Read the model definition and answer for the solid it produces. Units are mm, in the model's axes. Face numbers are marked on the shaded views. Round coordinates to 2 decimals unless told otherwise and drop trailing zeros. Order: outer loops, then holes, each group sorted by start corner. A loop starts at its lowest first (then second) coordinate and runs counter-clockwise, first axis right, second up. Notation, with made-up numbers: (74, -18) - (105, -18) arc R12 cw to (105, -2) - close; hole circle Ø4 at (58, 79). An arc over 180 degrees is marked (long way). Put each result on its own line as item: value. Start each with the question number.
Q1. Find the intervals of material crossed by line 1 along Y through (x, z) = (18.75, 2.5); line 2 along Z through (x, y) = (14, 0); line 3 along X through (y, z) = (-17, 2.25), in increasing order. Write a range as from..to.
Q2. For a pull along Z with two mould halves and no side action, classify the marked faces 1, 2 and 3 as pulls with the +Z half, pulls with the -Z half, needs draft (parallel to the pull), parting line crosses it, or undercut.
Q3. Section B-B on y = -2 is taken. Give the vertices of the cut face in (x, z).
Q4. Each of these flat-tipped pins is pushed along its axis until it touches: pin 1 Ø3 at (y, z) = (19.5, 2.5) entering from +X; pin 2 Ø1.5 at (y, z) = (-19.5, 2.5) entering from -X. Where does it stop, or does it pass through?
Q5. Section A-A on x = 14 is taken. Give the vertices of the cut face in (y, z), then the cut area to 4 significant figures.
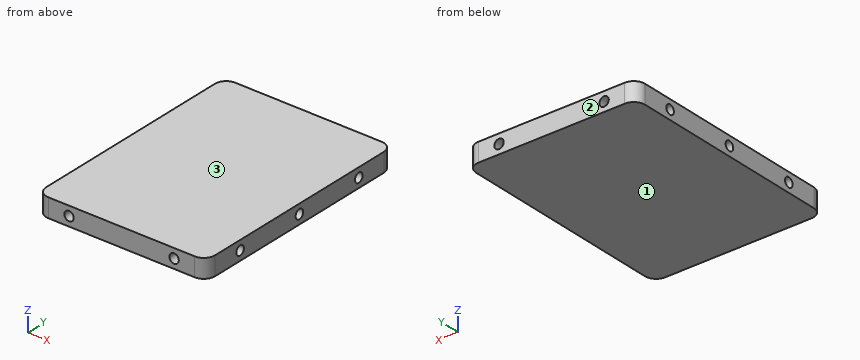
from build123d import *

# Parameters (mm, degrees)
SKETCH_1_W         = 45
SKETCH_1_H         = 61.4
EXTRUDE_1_DEPTH    = 5
HOLE_WIZARD_M3_3_D = 2.5
HOLE_WIZARD_M3_4_D = 2.5
FILLET_1_R         = 3


with BuildPart() as part:
    # 草图1 → 凸台-拉伸1 (new body)
    with BuildSketch(Plane.XY):
        Rectangle(SKETCH_1_W, SKETCH_1_H)
    extrude(amount=EXTRUDE_1_DEPTH)

    # 草图3 → M3 螺纹孔1 (revolve, cut)
    with BuildSketch(Plane(origin=(-22.5, 0, 2.5), x_dir=(0, 0, 1), z_dir=(0, 1, 0))):
        Polygon((0, 0), (0, 5.751075774), (1.25, 5), (1.25, 0), align=None)
    hole_wizard_m3_1 = revolve(axis=Axis((-28.85, 0, 2.5), (1, 0, 0)), mode=Mode.SUBTRACT)

    # 草图5 → M3 螺纹孔2 (revolve, cut)
    with BuildSketch(Plane(origin=(-22.5, 19.5, 2.5), x_dir=(0, 0, 1), z_dir=(0, 1, 0))):
        Polygon((0, 0), (0, 5.751075774), (1.25, 5), (1.25, 0), align=None)
    hole_wizard_m3_2 = revolve(axis=Axis((-28.85, 19.5, 2.5), (1, 0, 0)), mode=Mode.SUBTRACT)

    # 镜向1: M3 螺纹孔2 across plane
    add(hole_wizard_m3_2.mirror(Plane.ZX), mode=Mode.SUBTRACT)

    # M3 螺纹孔3 (through all)
    with Locations(Plane(origin=(0, -30.7, 0), x_dir=(-1, 0, 0), z_dir=(0, -1, 0))):
        with Locations((-14, -2.5)):
            hole_wizard_m3_3 = Hole(HOLE_WIZARD_M3_3_D / 2)

    # 镜向2: M3 螺纹孔3 across plane
    add(hole_wizard_m3_3.mirror(Plane(origin=(0, 0, 0), x_dir=(0, 0, 1), z_dir=(1, 0, 0))), mode=Mode.SUBTRACT)

    # 镜向3: M3 螺纹孔2, M3 螺纹孔1 across plane
    add(hole_wizard_m3_2.mirror(Plane(origin=(0, 0, 0), x_dir=(0, 0, 1), z_dir=(1, 0, 0))), mode=Mode.SUBTRACT)
    add(hole_wizard_m3_1.mirror(Plane(origin=(0, 0, 0), x_dir=(0, 0, 1), z_dir=(1, 0, 0))), mode=Mode.SUBTRACT)

    # 镜向3 copy 1 sketch → 镜向3 copy 1 (revolve, cut)
    with BuildSketch(Plane(origin=(22.5, -19.5, 2.5), x_dir=(0, 0, 1), z_dir=(0, -1, 0))):
        Polygon((0, 0), (0, 5.751075774), (1.25, 5), (1.25, 0), align=None)
    revolve(axis=Axis((28.85, -19.5, 2.5), (-1, 0, 0)), mode=Mode.SUBTRACT)

    # M3 螺纹孔4 (through all)
    with Locations(Plane(origin=(0, 30.7, 0), x_dir=(1, 0, 0), z_dir=(0, 1, 0))):
        with Locations((-14, -2.5), (14, -2.5)):
            Hole(HOLE_WIZARD_M3_4_D / 2)

    # 圆角1
    fillet_1_edges = [part.edges().sort_by_distance(p)[0] for p in [
        (22.5, -30.7, 2.5),
        (-22.5, -30.7, 2.5),
        (-22.5, 30.7, 2.5),
        (22.5, 30.7, 2.5),
    ]]
    fillet(fillet_1_edges, radius=FILLET_1_R)


solid = part.part
Findings:
1. line 1: -30.7..-20.75, -18.25..-1.25, 1.25..18.25, 20.75..30.7
1. line 2: 0..1.25, 3.75..5
1. line 3: -22.5..-15.22, -12.78..12.78, 15.22..22.5
2. face 1: pulls with the -Z half
2. face 2: needs draft
2. face 3: pulls with the +Z half
3. outline: (-22.5, 0) - (22.5, 0) - (22.5, 5) - (-22.5, 5) - close; hole circle Ø2.5 at (-14, 2.5); hole circle Ø2.5 at (14, 2.5)
4. pin 1: x = 22.5
4. pin 2: x = -17.2
5. outline: (-30.7, 0) - (30.7, 0) - (30.7, 1.25) - (-30.7, 1.25) - close; (-30.7, 3.75) - (30.7, 3.75) - (30.7, 5) - (-30.7, 5) - close
5. area: 153.5 mm2
